Check sheet for the modelled part. Datum: model origin and axes. Units: mm. Face numbers are marked on the shaded views. A direction names the side the tool comes from. Give positions to 0.01 mm unless a question says otherwise; leave off trailing zeros. Order: outer loops, then holes, each group sorted by start corner. A loop starts at its lowest first (then second) coordinate and runs counter-clockwise, first axis right, second up.
Item 1: Sectioned sample at C-C on y = -7.5. Record the boundary of the cut face in (x, z), and give its area (3 significant figures).
Item 2: Access from +Z, -Z, +X, -X, +Y, -Y to the whole of each face (thin tool, end or side, straight path). Record for the marked faces 1 and 2.
Item 3: Sectioned sample at A-A on y = 4.5. Record the boundary of the cut face in (x, z).
Item 4: Sectioned sample at B-B on z = 0. Record the boundary of the cut face in (x, y), and give its area (3 significant figures).
Item 5: Material ranges on line 1 along X through (y, z) = (-6.25, 0); line 2 along Y through (x, z) = (-1, -2); line 3 along X through (y, z) = (3.1, 0), recorded low to high.
Item 6: Sectioned sample at D-D on y = -3. Record the boundary of the cut face in (x, z), and give its area (3 significant figures).
Item 7: Gauge pin test, flat ends, axial feed: P1, Ø1.5, axis at y = -3.5, z = 1.5, coming from the +X side; P2, Ø4, axis at y = 0, z = 4, coming from the -X side; P3, Ø1.5, axis at x = 2.5, y = -2, coming from the +Z side. Record the tip position at first contact, or that the pin passes through.
Item 8: Release check for a two-part mould opening along Z. For the marked faces 3, 4 and 5 record: released by +Z, released by -Z, zero draft, split by the parting line, or undercut.
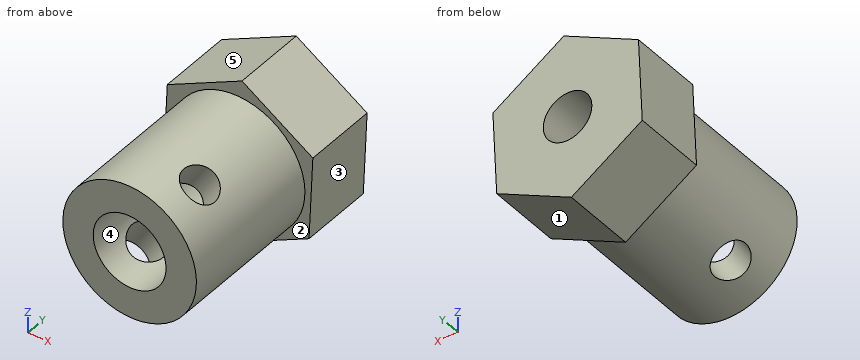
from build123d import *

# Parameters (mm, degrees)
SKETCH_1_R          = 2
EXTRUDE_1_DEPTH     = 6
SKETCH_1_3_R        = 5.5
SKETCH_1_3_R_2      = 3
EXTRUDE_2_DEPTH     = 12
SKETCH_2_R          = 1.5
CUT_EXTRUDE_1_DEPTH = 30


with BuildPart() as part:
    # Sketch 1 → Extrude 1 (new body)
    with BuildSketch(Plane(origin=(0, 0, 0), x_dir=(1, 0, 0), z_dir=(0, 1, 0))):
        Polygon((5.837094583, 3.732067367), (-0.313517857, 6.921105876), (-6.15061244, 3.18903851), (-5.837094583, -3.732067367), (0.313517857, -6.921105876), (6.15061244, -3.18903851), align=None)
        with Locations(Location((0, 0, 0), (0, 0, 270))):
            Circle(SKETCH_1_R, mode=Mode.SUBTRACT)
    extrude(amount=EXTRUDE_1_DEPTH)

    # Sketch 1_3 → Extrude 2 (add)
    with BuildSketch(Plane(origin=(0, 0, 0), x_dir=(1, 0, 0), z_dir=(0, 1, 0))):
        with Locations(Location((0, 0, 0), (0, 0, 270))):
            Circle(SKETCH_1_3_R)
        with Locations(Location((0, 0, 0), (0, 0, 270))):
            Circle(SKETCH_1_3_R_2, mode=Mode.SUBTRACT)
    extrude(amount=-EXTRUDE_2_DEPTH)

    # Sketch 2 → Cut-Extrude 1 (cut)
    with BuildSketch(Plane(origin=(3.232065148, 0, 5.055072193), x_dir=(0.8425120321737304, 0, -0.5386775247237361), z_dir=(0.538677524723736, 0, 0.8425120321737303))):
        with Locations((0, -8.135313369)):
            Circle(SKETCH_2_R)
    extrude(amount=-CUT_EXTRUDE_1_DEPTH, mode=Mode.SUBTRACT)


solid = part.part
Report:
1. outline: (-4.02, -3.76) - (-2.59, -1.52) arc R3 cw to (0.3, 2.99) - (1.73, 5.22) arc R5.5 ccw to start; (-1.73, -5.22) arc R5.5 ccw to (4.02, 3.76) - (2.59, 1.52) arc R3 cw to (-0.3, -2.99) - close
1. area: 52.9 mm2
2. face 1: -Z, +X, +Y, -Y
2. face 2: -Y
3. outline: (-6.15, -3.19) - (-0.31, -6.92) - (5.84, -3.73) - (6.15, 3.19) - (0.31, 6.92) - (-5.84, 3.73) - close; hole circle Ø4 at (0, 0)
4. outline: (-6.01, 0) - (-5.5, 0) - (-5.5, -12) - (-3, -12) - (-3, 0) - (-2, 0) - (-2, 6) - (-6.01, 6) - close; (2, 0) - (3, 0) - (3, -12) - (5.5, -12) - (5.5, 0) - (6.01, 0) - (6.01, 6) - (2, 6) - close
4. area: 108 mm2
5. line 1: x = -5.5 to -3, 3 to 5.5
5. line 2: y = 0 to 6
5. line 3: x = -6.01 to -2, 2 to 6.01
6. outline: circle Ø11 at (0, 0); hole circle Ø6 at (0, 0)
6. area: 66.8 mm2
7. P1: stops at x = 5.45
7. P2: stops at x = -5.92
7. P3: stops at z = 5.21
8. face 3: released by -Z
8. face 4: undercut
8. face 5: released by +Z
